Autodesk Inventor part; units mm, degrees
ref_plane "Work Plane2" through (3, -5, 1.9) normal (0, 0, 1) x (1, 0, 0)
ref_plane "Work Plane4" through (9.5, -2, 4.9) normal (0, 0, 1) x (1, 0, 0)
ref_plane "Work Plane6" through (-0.3541, -8.3541, 13) normal (0, 0, 1) x (1, 0, 0)
ref_plane "Work Plane1" through (0, 0, 0) normal (0, 0, 1) x (1, 0, 0)
sketch "Sketch1" plane through (0, 0, 0) normal (0, 0, 1) x (1, 0, 0)
  circle A0 centre (8, 0) radius 5 construction
  circle A1 centre (0, 18) radius 2 construction
  circle A2 centre (0, -18) radius 2 construction
  arc A3 (-10.2835, -9.5) -> (-3, -13.6748) centre (0, 0) ccw construction
  line L0 (-3, -13.6748) -> (-3, -18) construction
  arc A4 (-3, -18) -> (3, -18) centre (0, -18) ccw construction
  line L1 (3, -18) -> (3, -13.6748) construction
  arc A5 (3, -13.6748) -> (3, 13.6748) centre (0, 0) ccw construction
  line L2 (3, 13.6748) -> (3, 18) construction
  arc A6 (3, 18) -> (-3, 18) centre (0, 18) ccw construction
  line L3 (-3, 18) -> (-3, 13.6748) construction
  arc A7 (-3, 13.6748) -> (-10.2835, 9.5) centre (0, 0) ccw construction
  line L4 (-10.2835, 9.5) -> (-15.2835, 9.5) construction
  line L5 (-15.2835, 9.5) -> (-15.2835, -9.5) construction
  line L6 (-15.2835, -9.5) -> (-10.2835, -9.5) construction
  circle A8 centre (8, 0) radius 5.2
  circle A9 centre (0, -18) radius 1.7
  circle A10 centre (0, 18) radius 1.7
  line L7 (8, 0) -> (0, 0) construction
  line L8 (8, 0) -> (0, 0)
  line L9 (18.2, 24.7) -> (-6.7, 24.7)
  line L10 (-6.7, 24.7) -> (-6.7, -24.7)
  line L11 (-6.7, -24.7) -> (18.2, -24.7)
  line L12 (18.2, -24.7) -> (18.2, 24.7)
  point P0 (13.2, 0)
  point P1 (-1.7, 18)
  point P2 (0, 19.7)
  dimension "d0" = 0.2
  dimension "d3" = 5
  dimension "d4" = 5
  dimension "d5" = 5
  dimension "d20" = 3.4
ref_plane "Work Plane2" through (3, -5, 1.9) normal (0, 0, 1) x (1, 0, 0)
ref_plane "Work Plane3" through (8, 0, 2) normal (0, 0, 1) x (1, 0, 0)
extrude "Extrusion1" add sketch "Sketch1" along normal up to surface (2 mm away)
sketch "Sketch2" plane through (-6.7, 24.7, 2) normal (0, 0, 1) x (1, 0, 0)
  circle A0 centre (6.7, -6.7) radius 1.7
  circle A1 centre (6.7, -42.7) radius 1.7
  circle A2 centre (14.7, -24.7) radius 5.2 construction
  line L0 (0, 0) -> (24.9, 0)
  line L1 (0, -49.4) -> (0, 0)
  line L2 (24.9, -49.4) -> (0, -49.4)
  line L3 (24.9, 0) -> (24.9, -49.4)
  circle A3 centre (14.7, -24.7) radius 2.5 construction
  circle A4 centre (14.7, -24.7) radius 2.7
  point P0 (6.7, -24.7)
  dimension "d8" = 0.2
ref_plane "Work Plane4" through (9.5, -2, 4.9) normal (0, 0, 1) x (1, 0, 0)
extrude "Extrusion2" add sketch "Sketch2" along normal up to surface (2.9 mm away)
sketch "Sketch3" plane through (-6.7, -24.7, 4.9) normal (0, 0, 1) x (1, 0, 0)
  arc A0 (18.0541, 25.7) -> (15.7, 28.0541) centre (14.7, 24.7) ccw construction
  line L0 (15.7, 33.0541) -> (15.7, 28.0541) construction
  line L1 (13.7, 33.0541) -> (15.7, 33.0541) construction
  line L2 (13.7, 28.0541) -> (13.7, 33.0541) construction
  arc A1 (13.7, 28.0541) -> (11.3459, 25.7) centre (14.7, 24.7) ccw construction
  line L3 (6.3459, 25.7) -> (11.3459, 25.7) construction
  line L4 (6.3459, 23.7) -> (6.3459, 25.7) construction
  line L5 (11.3459, 23.7) -> (6.3459, 23.7) construction
  arc A2 (11.3459, 23.7) -> (13.7, 21.3459) centre (14.7, 24.7) ccw construction
  line L6 (13.7, 16.3459) -> (13.7, 21.3459) construction
  line L7 (15.7, 16.3459) -> (13.7, 16.3459) construction
  line L8 (15.7, 21.3459) -> (15.7, 16.3459) construction
  arc A3 (15.7, 21.3459) -> (18.0541, 23.7) centre (14.7, 24.7) ccw construction
  line L9 (23.0541, 23.7) -> (18.0541, 23.7) construction
  line L10 (23.0541, 25.7) -> (23.0541, 23.7) construction
  line L11 (18.0541, 25.7) -> (23.0541, 25.7) construction
  circle A4 centre (14.7, 24.7) radius 8.4137 construction
  arc A5 (17.9486, 32.5696) -> (17.9486, 16.8304) centre (14.7, 24.7) ccw
  circle A6 centre (6.7, 42.7) radius 1.7
  circle A7 centre (6.7, 6.7) radius 1.7
  circle A8 centre (14.7, 24.7) radius 2.7
  line L12 (0, 0) -> (0, 49.4)
  line L13 (24.9, 0) -> (0, 0)
  line L14 (24.9, 49.4) -> (24.9, 0)
  line L15 (0, 49.4) -> (24.9, 49.4)
  line L16 (0, 49.4) -> (0, 0)
  circle A9 centre (14.7, 24.7) radius 2.7
  line L17 (14.7, 24.7) -> (0, 24.7) construction
  line L18 (17.9486, 16.8304) -> (24.9, 19.7)
  line L19 (24.9, 0) -> (24.9, 49.4)
  line L20 (17.9486, 32.5696) -> (24.9, 29.7)
  line L21 (13.7, 16.2452) -> (0, 11.7)
  line L22 (13.7, 33.1548) -> (0, 37.7)
  point P0 (6.7, 24.7)
  point P1 (0, 37.7)
  point P2 (24.9, 19.7)
  point P3 (0, 11.7)
  point P4 (0, 37.7)
  dimension "d11" = 0.1
  dimension "d13" = 10
  dimension "d17" = 5
ref_plane "Work Plane5" through (8, 0, 13.1) normal (0, 0, 1) x (-1, 0, 0)
ref_plane "Work Plane6" through (-0.3541, -8.3541, 13) normal (0, 0, 1) x (1, 0, 0)
extrude "Extrusion3" add sketch "Sketch3" along normal up to surface (8.1 mm away) contours A5 L22 L12 L15 L14 L20 | A5 L18 L14 L13 L12 L21
sketch "Sketch4" plane through (-6.7, -24.7, 0) normal (-1, 0, 0) x (0, 0, 1)
  line L0 (0, 49.4) -> (13, 49.4)
  line L1 (0, 49.4) -> (0, 0)
  line L2 (0, 0) -> (13, 0)
  line L3 (13, 0) -> (13, 11.7)
  line L4 (4.9, 11.7) -> (13, 11.7)
  line L5 (4.9, 11.7) -> (4.9, 37.7)
  line L6 (4.9, 37.7) -> (13, 37.7)
  line L7 (13, 37.7) -> (13, 49.4)
  point P0 (0, 24.7)
extrude "Extrusion4" add sketch "Sketch4" along normal blind 20
sketch "Sketch5" plane through (18.2, -24.7, 13) normal (0, 0, 1) x (1, 0, 0)
  circle A0 centre (-18.2, 6.7) radius 1.7
  circle A1 centre (-18.2, 6.7) radius 1.7
  line L0 (0, 0) -> (-44.9, 0)
  circle A2 centre (-28.2, 6.7) radius 1.7
  circle A3 centre (-38.2, 6.7) radius 1.7
  circle A4 centre (-8.2, 6.7) radius 1.7
  circle A5 centre (-18.2, 6.7) radius 1.7
  circle A6 centre (-28.2, 6.7) radius 1.7
  point P0 (-18.2, 24.7)
  dimension "d23" = 10
  dimension "d26" = 10
extrude "Extrusion5" cut sketch "Sketch5" against normal through all contours A2 | A3 | A4
mirror "Mirror1" about plane through (0, 0, 0) normal (0, 1, 0) of "Extrusion5"
sketch "Sketch6" plane through (18.2, -24.7, 0) normal (1, 0, 0) x (0, 0, -1)
  line L0 (0, 0) -> (-13, 0)
  line L1 (0, 0) -> (0, 49.4)
  line L2 (0, 49.4) -> (-13, 49.4)
  line L3 (-13, 49.4) -> (-13, 29.7)
  line L4 (-4.9, 29.7) -> (-13, 29.7)
  line L5 (-4.9, 29.7) -> (-4.9, 19.7)
  line L6 (-4.9, 19.7) -> (-13, 19.7)
  line L7 (-13, 19.7) -> (-13, 0)
  line L8 (-11, 31.7) -> (-11, 47.4)
  line L9 (-11, 47.4) -> (-2, 47.4)
  line L10 (-2, 47.4) -> (-2, 2)
  line L11 (-2, 2) -> (-11, 2)
  line L12 (-11, 2) -> (-11, 17.7)
  line L13 (-11, 17.7) -> (-2.9, 17.7)
  line L14 (-2.9, 17.7) -> (-2.9, 31.7)
  line L15 (-2.9, 31.7) -> (-11, 31.7)
  line L16 (-11, 31.7) -> (-13, 31.7)
  line L17 (-13, 49.4) -> (-13, 29.7)
  line L18 (-11, 17.7) -> (-13, 17.7)
  point P0 (0, 24.7)
  point P1 (-13, 31.7)
  dimension "d31" = 2
ref_plane "Work Plane7" through (36.9, -26.2379, 21.2621) normal (1, 0, 0) x (0, 0.9775, 0.2109)
extrude "Extrusion6" add sketch "Sketch6" along normal up to surface (18.7 mm away) contours L7 L6 L5 L4 L3 L16 L15 L14 L13 L18
The model under review builds one solid part; all positions refer to its coordinate system, in mm. A direction names the side the tool comes from. Give positions to 0.01 mm unless a question says otherwise; leave off trailing zeros. Write each loop counter-clockwise with the first axis right and the second up, starting at its lowest first coordinate (ties: lowest second). Pieces come first, ordered by that corner, then holes. Notation, with made-up numbers: M 58,51.5 L 89,51.5 A17 cw 89,70.5 Z; hole C 14.5,-11.5 d8. An arc over 180 degrees is marked long. Answer in a Markdown table with one row per item.
Item 1: For line 1 along Y through (x, z) = (-10, 9.75); line 2 along Y through (x, z) = (-10, 4); line 3 along Y through (x, z) = (0, 9.5), list the stretches that pass through material, from the lowest coordinate up.
Check sheet entries:
| item | result |
|---|---|
| line 1 | -24.7 to -19.7, -16.3 to -13, 13 to 16.3, 19.7 to 24.7 |
| line 2 | -24.7 to -19.7, -16.3 to 16.3, 19.7 to 24.7 |
| line 3 | -24.7 to -19.7, -16.3 to -10.78, 10.78 to 16.3, 19.7 to 24.7 |
Item 2: For P1, Ø5.5, axis at x = -10, y = 18, coming from the +Z side; P2, Ø4, axis at x = -19.5, y = 6, coming from the +Z side; P3, Ø2.5, axis at x = 29.5, z = 10.5, coming from the -Y side; P4, Ø5, axis at x = 26.5, y = 8, coming from the -Z side, all flat-tipped, find the tip position at first contact; note any pin that passes through.
Check sheet entries:
| item | result |
|---|---|
| P1 | z = 13 |
| P2 | z = 4.9 |
| P3 | y = -7 |
| P4 | z = 2.9 |
Item 3: Add section D-D on x = 21.5. Give the boundary of the cut face in (y, z), plus the area to 3 significant figures.
Check sheet entries:
| item | result |
|---|---|
| outline | M -7,2.9 L 7,2.9 L 7,13 L 5,13 L 5,4.9 L -5,4.9 L -5,13 L -7,13 Z |
| area | 60.4 mm2 |
Item 4: Draft analysis for pull direction X (two halves, no side actions). For faces 1 (the face through (9.779, 19.686, 6.591)), 2 (the face through (0.246, 10.696, 8.893)), 3 (the face through (-2, 17, 13)), state which applies: +X half, -X half, draft (parallel to the pull), parting line (faces both ways), or undercut.
Check sheet entries:
| item | result |
|---|---|
| face 1 | undercut |
| face 2 | -X half |
| face 3 | draft |
Item 5: Add section B-B on x = -10. Give the boundary of the cut face in (y, z), plus the area to 3 significant figures.
Check sheet entries:
| item | result |
|---|---|
| outline | M -24.7,0 L -19.7,0 L -19.7,13 L -24.7,13 Z; M -16.3,0 L 16.3,0 L 16.3,13 L 13,13 L 13,4.9 L -13,4.9 L -13,13 L -16.3,13 Z; M 19.7,0 L 24.7,0 L 24.7,13 L 19.7,13 Z |
| area | 343 mm2 |
Item 6: Tool access review of faces 4 (the face through (-18.43, -18.65, 6.59)), 5 (the face through (10.2, -2.2, 2)), 6 (the face through (0.246, -10.696, 8.893)), 7 (the face through (9.19, -8.43, 8.89)), 8 (the face through (27, -5, 9)): name each direction out of +Z, -Z, +X, -X, +Y, -Y from which nothing blocks a thin tool from reaching the whole face with its end or side.
Check sheet entries:
| item | result |
|---|---|
| face 4 | +Z, -Z |
| face 5 | -Z |
| face 6 | +Z, -X |
| face 7 | +Z |
| face 8 | +Z, +X, -X |
Item 7: Add section C-C on z = 11.5. State how many separate pieces and enclosed holes the cut face has, plus the area to 3 significant figures.
Check sheet entries:
| item | result |
|---|---|
| separate pieces | 2 |
| enclosed holes | 8 |
| area | 1,250 mm2 |
Item 8: Add section A-A on y = 18. Give the boundary of the cut face in (x, z).
Check sheet entries:
| item | result |
|---|---|
| outline | M -26.7,0 L -21.7,0 L -21.7,13 L -26.7,13 Z; M -18.3,0 L -11.7,0 L -11.7,13 L -18.3,13 Z; M -8.3,0 L -1.7,0 L -1.7,13 L -8.3,13 Z; M 1.7,0 L 8.3,0 L 8.3,13 L 1.7,13 Z; M 11.7,0 L 18.2,0 L 18.2,13 L 11.7,13 Z |
